Design review of the part shown in the three views and the two pictorial views. Dimensions are in mm from the part's minimum x, y and z. A direction names the side the tool comes from. Coordinates: 2 decimals unless noted, no trailing zeros. Loops run counter-clockwise (first coordinate to the right, second up) from the corner with the lowest first, then second, coordinate; pieces in that order, holes last. Notation, with made-up numbers: (-5.5, 67) -> (29.5, 67) arc R21 cw to (29.5, 71) -> close; hole circle Ø10 at (-14.5, 52). An arc over 180 degrees is marked (long way). One line per item, written item: value.
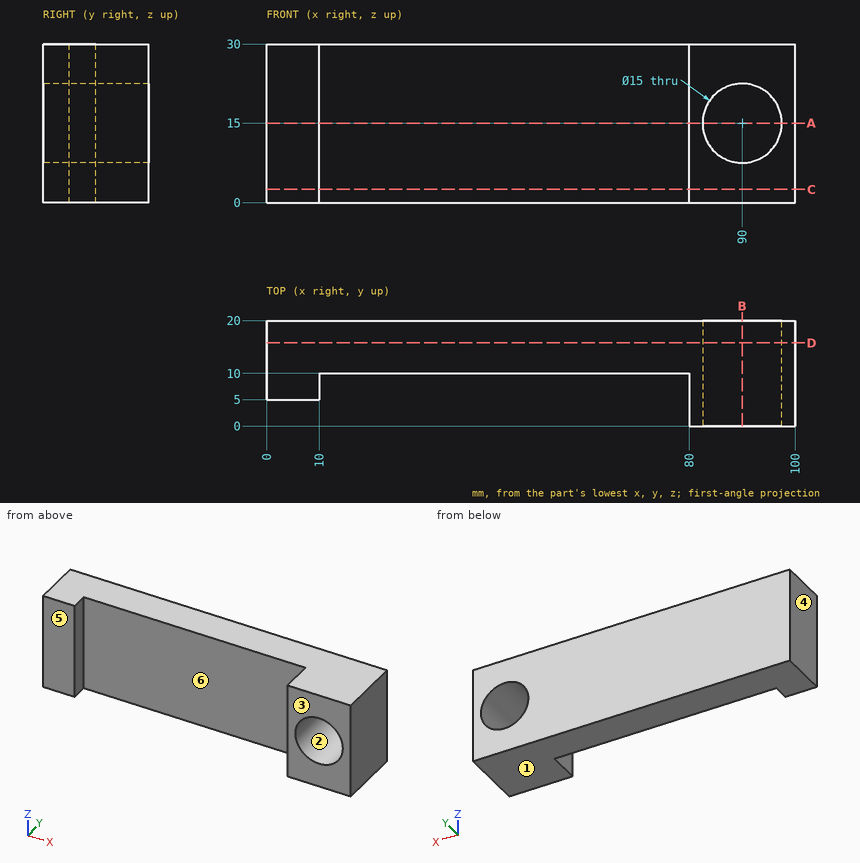
1. Take a section at B-B, the plane x = 90. Give the boundary of the cut face in (y, z).
Return value:
outline: (0, 0) -> (20, 0) -> (20, 7.5) -> (0, 7.5) -> close; (0, 22.5) -> (20, 22.5) -> (20, 30) -> (0, 30) -> close
2. Take a section at A-A, the plane z = 15. Give the boundary of the cut face in (x, y), and give its area (3 significant figures).
Return value:
outline: (0, 5) -> (10, 5) -> (10, 10) -> (80, 10) -> (80, 0) -> (82.5, 0) -> (82.5, 20) -> (0, 20) -> close; (97.5, 0) -> (100, 0) -> (100, 20) -> (97.5, 20) -> close
area: 950 mm2
3. For the marked faces 4, 5 and 6, list the 3-axis set-ups (+Z, -Z, +X, -X, +Y, -Y) from which the entire face can be reached by the end or side of a thin tool; tool diameter is ignored.
Return value:
face 4: +Z, -Z, -X, +Y, -Y
face 5: +Z, -Z, -X, -Y
face 6: +Z, -Z, -Y
4. The part is to be moulded in two halves that separate along Z. For the marked faces 1, 2 and 3, say which applies: pulls with the +Z half, pulls with the -Z half, needs draft (parallel to the pull), parting line crosses it, or undercut.
Return value:
face 1: pulls with the -Z half
face 2: undercut
face 3: needs draft
5. Insertion check: pin 1 Ø8 at (x, z) = (29.5, 22.5) entering from -Y; pin 2 Ø13.5 at (x, z) = (90, 15) entering from +Y; pin 3 Ø8 at (y, z) = (7, 14.5) entering from -X; pin 4 Ø3 at (x, z) = (6, 11) entering from -Y. Each pin has a flat end and moves straight along its axis. Give the tip position at first contact, or say it passes through.
Return value:
pin 1: stops at y = 10
pin 2: passes through
pin 3: stops at x = 0
pin 4: stops at y = 5
6. To check wall thickness, follow probe 1 along X at (y, z) = (6.25, 25.5); probe 2 along Z at (x, y) = (89.5, 3.5); probe 3 along X at (y, z) = (6.75, 13.5). State the ranges of each line that lie inside material, in increasing order. Write a range as from..to.
Return value:
probe 1: x = 0..10, 80..100
probe 2: z = 0..7.52, 22.48..30
probe 3: x = 0..10, 80..82.65, 97.35..100
7. Take a section at C-C, the plane z = 2.5. Give the boundary of the cut face in (x, y), and give its area (3 significant figures).
Return value:
outline: (0, 5) -> (10, 5) -> (10, 10) -> (80, 10) -> (80, 0) -> (100, 0) -> (100, 20) -> (0, 20) -> close
area: 1,250 mm2
8. Take a section at D-D, the plane y = 15.75. Give the boundary of the cut face in (x, z), and give its area (3 significant figures).
Return value:
outline: (0, 0) -> (100, 0) -> (100, 30) -> (0, 30) -> close; hole circle Ø15 at (90, 15)
area: 2,820 mm2
